Autodesk Inventor part; units mm, degrees
ref_plane "YZ Plane" through (0, 0, 0) normal (1, 0, 0) x (0, 1, 0)
ref_plane "XZ Plane" through (0, 0, 0) normal (0, 1, 0) x (-1, 0, 0)
ref_plane "XY Plane" through (0, 0, 0) normal (0, 0, 1) x (1, 0, 0)
sketch "Sketch1" plane through (0, 0, 0) normal (0, 0, 1) x (1, 0, 0)
  circle A0 centre (0, 0) radius 43.5
  circle A1 centre (0, 35) radius 2.6
  circle A2 centre (-13.3939, 32.3358) radius 2.6
  circle A3 centre (-24.7487, 24.7487) radius 2.6
  circle A4 centre (-32.3358, 13.3939) radius 2.6
  circle A5 centre (-35, 0) radius 2.6
  circle A6 centre (-32.3358, -13.3939) radius 2.6
  circle A7 centre (-24.7487, -24.7487) radius 2.6
  circle A8 centre (-13.3939, -32.3358) radius 2.6
  circle A9 centre (0, -35) radius 2.6
  circle A10 centre (13.3939, -32.3358) radius 2.6
  circle A11 centre (24.7487, -24.7487) radius 2.6
  circle A12 centre (32.3358, -13.3939) radius 2.6
  circle A13 centre (35, 0) radius 2.6
  circle A14 centre (32.3358, 13.3939) radius 2.6
  circle A15 centre (24.7487, 24.7487) radius 2.6
  circle A16 centre (13.3939, 32.3358) radius 2.6
  line L0 (0, 0) -> (0, -92.2535) construction
  line L1 (-9.7254, 0) -> (-9.7254, -92.2535)
  line L2 (9.7254, -92.2535) -> (9.7254, 0)
  arc A17 (9.7254, 0) -> (-9.7254, 0) centre (0, 0) ccw
  arc A18 (-9.7254, -92.2535) -> (9.7254, -92.2535) centre (0, -92.2535) ccw
  line L3 (0, 0) -> (-60.6432, 72.2718) construction
  line L4 (-7.6604, -6.4279) -> (-68.3037, 65.8439)
  line L5 (-52.9828, 78.6997) -> (7.6604, 6.4279)
  arc A19 (-7.6604, -6.4279) -> (7.6604, 6.4279) centre (0, 0) ccw
  arc A20 (-52.9828, 78.6997) -> (-68.3037, 65.8439) centre (-60.6432, 72.2718) ccw
  line L6 (0, 0) -> (65.9097, 78.5481) construction
  line L7 (-7.6604, 6.4279) -> (58.2493, 84.976)
  line L8 (73.5702, 72.1203) -> (7.6604, -6.4279)
  arc A21 (-7.6604, 6.4279) -> (7.6604, -6.4279) centre (0, 0) ccw
  arc A22 (73.5702, 72.1203) -> (58.2493, 84.976) centre (65.9097, 78.5481) ccw
  circle A23 centre (0, 0) radius 20
  point P0 (0, -46.1267)
  point P1 (-30.3216, 36.1359)
  point P2 (32.9549, 39.2741)
  point P3 (18.7939, 6.8404)
  point P4 (3.473, 19.6962)
  point P5 (19.552, 38.8583)
  point P6 (-19.552, 38.8583)
  point P7 (-3.473, 19.6962)
  point P8 (-18.7939, 6.8404)
  point P9 (-34.8728, 26.0026)
  point P10 (-9.7254, -42.3989)
  point P11 (-9.7254, -17.4762)
  point P12 (9.7254, -17.4762)
  point P13 (9.7254, -42.3989)
  point P14 (34.8728, 26.0026)
  point P15 (7.6604, -6.4279)
  point P16 (9.7254, -3.9669)
  point P17 (-9.7254, -3.9669)
  dimension "d0" = 87
  dimension "d1" = 5.2
  dimension "d2" = 35
  dimension "d5" = 360
  dimension "d7" = 140
  dimension "d8" = 140
  dimension "d9" = 10
  dimension "d10" = 10
  dimension "d11" = 40
extrude "Extrusion1" add sketch "Sketch1" along normal blind 4 contours A0 L2 A23 L8 | L7 A16 A23 L5 A2 A0 | A23 L2 L8 | L8 L2 A19 L5 L7 A23 | A0 L4 A23 L1 | L7 A16 | L8 A19 L2 | L7 L5 A23 | A23 L4 L1 | A2 L5 | A19 A21 L1 A17 L2 | L2 A17 L1 A21 L7 L5 A19 | L7 A21 L1 L4 A23 L5 | L1 A21 L4 picked at (13.6821, 33.106) picked at (-12.7209, 31.8549)
sketch "Sketch2" plane through (0, 0, 0) normal (0, 0, -1) x (-1, 0, 0)
  circle A0 centre (0, 0) radius 7.65
  dimension "d14" = 15.3
extrude "Extrusion2" cut sketch "Sketch2" against normal blind 1.5
sketch "Sketch3" plane through (0, 0, 1.5) normal (0, 0, -1) x (-1, 0, 0)
  circle A0 centre (0, 0) radius 2.7
  dimension "d17" = 5.4
extrude "Extrusion3" cut sketch "Sketch3" against normal up to surface (2.5 mm away)
fillet "Fillet1" radius 4 12 edges at (9.7254, -3.9669, 2) (-9.7254, -3.9669, 2) (3.473, 19.6962, 2) (18.7939, 6.8404, 2) (-18.7939, 6.8404, 2) (-3.473, 19.6962, 2) (34.8728, 26.0026, 2) (19.552, 38.8583, 2) (-19.552, 38.8583, 2) (-34.8728, 26.0026, 2) (-9.7254, -42.3989, 2) (9.7254, -42.3989, 2)
equation "\"d10\" = d9"
properties part number "LED disk_3DPrint"
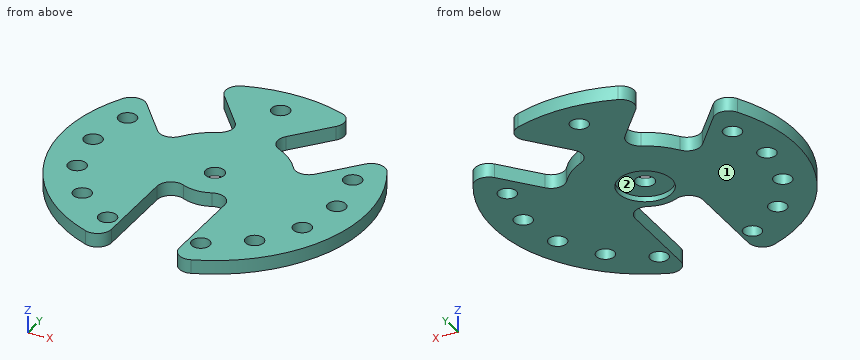
Source: CAD feature listing. Evaluate the final solid. Frame: model axes, mm. Face numbers are marked on the shaded views. Coordinates: 2 decimals unless noted, no trailing zeros. Order: outer loops, then holes, each group sorted by start corner. A loop starts at its lowest first (then second) coordinate and runs counter-clockwise, first axis right, second up.
Item 1: Cut plane A-A (x = 0). Return loops of the section in (y, z).
Output values:
outline: (-10, 0) - (-7.65, 0) - (-7.65, 1.5) - (-2.7, 1.5) - (-2.7, 4) - (-10, 4) - close; (2.7, 1.5) - (7.65, 1.5) - (7.65, 0) - (32.4, 0) - (32.4, 4) - (2.7, 4) - close; (37.6, 0) - (43.5, 0) - (43.5, 4) - (37.6, 4) - close
Item 2: Cut plane C-C (x = 24). Return loops of the section in (y, z).
Output values:
outline: (-36.28, 0) - (-27.24, 0) - (-27.24, 4) - (-36.28, 4) - close; (-22.26, 0) - (13.04, 0) - (13.04, 4) - (-22.26, 4) - close
Item 3: First-contact query: P1, Ø4, axis at x = 32.34, y = 13.39, coming from the -Z side; P2, Ø2, axis at x = -30, z = 3.5, coming from the -Y side; P3, Ø1, axis at x = -5, z = 0.5, coming from the +Y side; P4, Ø4.5, axis at x = 2, y = -2.5, coming from the -Z side. Flat tips, straight axial feed; report the tip coordinate or a pass-through.
Output values:
P1: passes through
P2: stops at y = -32.42
P3: stops at y = 43.27
P4: stops at z = 1.5
Item 4: Pull-direction query (X, two-part tool) for the marked faces 1 and 2; classes: pulls with the +X half, pulls with the -X half, needs draft (parallel to the pull), parting line crosses it, or undercut.
Output values:
face 1: needs draft
face 2: undercut
Item 5: Cut plane D-D (z = 3.35). Count the separate pieces of the cut face and the enclosed holes in it, plus the area to 3 significant figures.
Output values:
separate pieces: 1
enclosed holes: 12
area: 4,060 mm2
Item 6: Cut plane B-B (y = 0). Return loops of the section in (x, z).
Output values:
outline: (-43.5, 0) - (-37.6, 0) - (-37.6, 4) - (-43.5, 4) - close; (-32.4, 0) - (-7.65, 0) - (-7.65, 1.5) - (-2.7, 1.5) - (-2.7, 4) - (-32.4, 4) - close; (2.7, 1.5) - (7.65, 1.5) - (7.65, 0) - (32.4, 0) - (32.4, 4) - (2.7, 4) - close; (37.6, 0) - (43.5, 0) - (43.5, 4) - (37.6, 4) - close
Item 7: Material intervals for line 1 (Y direction, x = 0, z = 2.9); line 2 (Y direction, x = -13.5, z = 1.3); line 3 (X direction, y = -29, z = 2.2), sorted ascending.
Output values:
line 1: y = -10 to -2.7, 2.7 to 32.4, 37.6 to 43.5
line 2: y = -41.03 to -34.93, -29.74 to 14.76, 31.65 to 41.35
line 3: x = -32.42 to -9.73, 9.73 to 32.42
